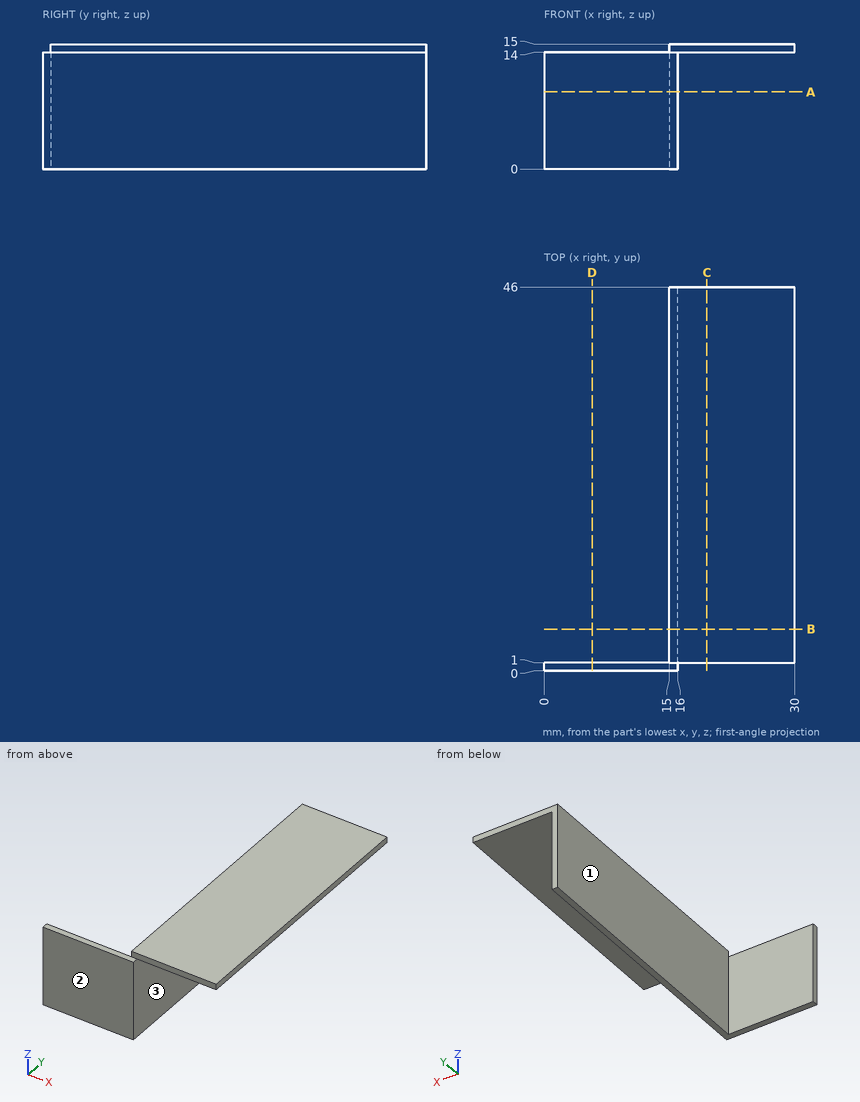
Here's the drawing with two shaded views (mm, measured from the low corner). I have some questions. A direction names the side the tool comes from. Give positions to 0.01 mm unless a question says otherwise; leave off trailing zeros. Write each loop counter-clockwise with the first axis right and the second up, starting at its lowest first coordinate (ties: lowest second). Pieces come first, ordered by that corner, then holes. Notation, with made-up numbers: (51, -7) -> (106, -7) arc R25 ccw to (106, 25) -> close; hole circle Ø8 at (67.5, -12). An arc over 180 degrees is marked (long way). Use one line per item in the form item = value.
1) Suppose I cut it at C-C (x = 19.5). Please give me the cut outline in (y, z), and give its area (3 significant figures).
Verdict:
outline = (1, 14) -> (46, 14) -> (46, 15) -> (1, 15) -> close
area = 45.0 mm2
2) I'm going to push flat-ended pins straight in: pin 1 (0.8 mm diameter, centred on x = 10.5, y = 0.5, fed in from +Z); pin 2 (0.5 mm diameter, centred on x = 22.5, z = 14.5, fed in from -Y); pin 3 (7.5 mm diameter, centred on y = 30.5, z = 11, fed in from -X); pin 4 (12 mm diameter, centred on x = 4, y = 9, fed in from -Z). Where does each tip first touch, or does it pass through?
Verdict:
pin_1 = 14
pin_2 = 1
pin_3 = 15
pin_4 = through
3) Suppose I cut it at A-A (z = 9.25). Please give me the cut outline in (x, y).
Verdict:
outline = (0, 0) -> (16, 0) -> (16, 46) -> (15, 46) -> (15, 1) -> (0, 1) -> close
4) If I drill on L1, parallel to X at y = 22, z = 11.25; L2, parallel to Z at x = 20.5, y = 22; L3, parallel to Y at x = 12.75, z = 12.5, over which ranges is the centre line in solid material (lowest first)? Write a range as [from, to].
Verdict:
L1 = [15, 16]
L2 = [14, 15]
L3 = [0, 1]
5) Suppose I cut it at B-B (y = 5). Please give me the cut outline in (x, z).
Verdict:
outline = (15, 0) -> (16, 0) -> (16, 14) -> (30, 14) -> (30, 15) -> (15, 15) -> close
6) Suppose I cut it at D-D (x = 5.75). Please give me the cut outline in (y, z).
Verdict:
outline = (0, 0) -> (1, 0) -> (1, 14) -> (0, 14) -> close
7) On a 3-axis mill with a long thin cutter (end or side, diameter ignored), from which of +Z, -Z, +X, -X, +Y, -Y can I reach the whole of each face in a straight line? I mean the marked faces 1, 2 and 3. Say none if no direction works.
Verdict:
face_1 = +Z, -Z, -X, +Y
face_2 = +Z, -Z, +X, -X, -Y
face_3 = -Z, +X, +Y, -Y
